CAD build for the part. Positions are in the model's coordinates, mm. A direction names the side the tool comes from. Give positions to 0.01 mm unless a question says otherwise; leave off trailing zeros. Write each loop counter-clockwise with the first axis right and the second up, starting at its lowest first coordinate (ties: lowest second). Pieces come first, ordered by that corner, then holes. Notation, with made-up numbers: (2, 18) - (9, 18) arc R26 ccw to (9, 38) - close; hole circle Ø6 at (0, 85.5). An arc over 180 degrees is marked (long way). Answer as a JSON object with one key per item and string values.
Autodesk Inventor part; units mm, degrees
ref_plane "YZ Plane" through (0, 0, 0) normal (1, 0, 0) x (0, 1, 0)
ref_plane "XZ Plane" through (0, 0, 0) normal (0, 1, 0) x (-1, 0, 0)
ref_plane "XY Plane" through (0, 0, 0) normal (0, 0, 1) x (1, 0, 0)
sketch "Sketch1" plane through (0, 0, 0) normal (0, 1, 0) x (-1, 0, 0)
  line L0 (86.0424, 26.9023) -> (56.0424, 26.9023)
  line L1 (2.5, 83.15) -> (-2.5, 83.15)
  line L2 (2.5, 83.15) -> (2.5, 73.15)
  line L3 (-2.5, 83.15) -> (-2.5, 73.15)
  circle A0 centre (0, 0) radius 90.15
  line L4 (-86.0424, 26.9023) -> (-56.0424, 26.9023)
  line L5 (-56.0424, 26.9023) -> (-56.0424, 36.9023)
  line L6 (-56.0424, 36.9023) -> (-66.0424, 36.9023)
  line L7 (56.0424, 26.9023) -> (56.0424, 36.9023)
  line L8 (56.0424, 36.9023) -> (66.0424, 36.9023)
  line L9 (-17.9658, 43.15) -> (-2.5, 73.15)
  line L10 (17.5, 43.15) -> (2.5, 73.15)
  line L11 (17.5, 43.15) -> (26.4443, 47.6221)
  line L12 (26.4443, 47.6221) -> (13.6803, 73.15)
  line L13 (-17.9658, 43.15) -> (-26.9101, 47.6221)
  line L14 (-26.9101, 47.6221) -> (-13.7498, 73.15)
  arc A1 (66.0424, 36.9023) -> (13.6803, 73.15) centre (4.3796, 3.7706) ccw
  arc A2 (-13.7498, 73.15) -> (-66.0424, 36.9023) centre (-4.3742, 3.7807) ccw
  dimension "d28" = 180.3
  dimension "d1" = 30
  dimension "d20" = 5
  dimension "d21" = 10
  dimension "d22" = 10
  dimension "d29" = 30
  dimension "d30" = 10
  dimension "d31" = 10
  dimension "d32" = 10
  dimension "d33" = 10
  dimension "d37" = 10
  dimension "d38" = 10
  dimension "d39" = 70
  dimension "d40" = 70
extrude "Extrusion1" add sketch "Sketch1" along normal blind 7 contours L0 L7 L8 A1 L12 L11 L10 L2 L1 L3 L9 L13 L14 A2 L6 L5 L4 A0 picked at (-11.4052, 63.15)
sketch "Sketch2" plane through (0, 0, 0) normal (0, -1, 0) x (1, 0, 0)
  circle A0 centre (74.2273, 36.5899) radius 3.35
  circle A1 centre (-74.0777, 36.5899) radius 3.35
  circle A2 centre (-13.319, 81.4854) radius 3.35
  circle A3 centre (13.1694, 81.4854) radius 3.35
  point P0 (0, 0)
  dimension "d43" = 6.7
  dimension "d44" = 6.7
  dimension "d45" = 6.7
  dimension "d46" = 6.7
extrude "Extrusion2" cut sketch "Sketch2" against normal blind 4.7
properties part number "Droplet Launcher 2"
Item 1: Cut at C-C (y = 3). Give the cut face in (x, z).
Entries:
{"outline": "(-86.04, 26.9) - (-56.04, 26.9) - (-56.04, 36.9) - (-66.04, 36.9) arc R70 cw to (-13.68, 73.15) - (-26.44, 47.62) - (-17.5, 43.15) - (-2.5, 73.15) - (-2.5, 83.15) - (2.5, 83.15) - (2.5, 73.15) - (17.97, 43.15) - (26.91, 47.62) - (13.75, 73.15) arc R70 cw to (66.04, 36.9) - (56.04, 36.9) - (56.04, 26.9) - (86.04, 26.9) arc R90.15 ccw to start; hole circle Ø6.7 at (-74.08, 36.59); hole circle Ø6.7 at (-13.32, 81.49); hole circle Ø6.7 at (13.17, 81.49); hole circle Ø6.7 at (74.23, 36.59)"}
Item 2: Probe line 1 (X direction, y = 5.25, z = 68.5) (3 decimals); line 2 (Z direction, x = -14, y = 1); line 3 (X direction, y = 6, z = 65) (3 decimals). List the from-to ranges inside material, lowest first. Write a range as from..to.
Entries:
{"line 1": "-58.607..-31.028, -16.005..-4.825, 4.897..16.147, 31.047..58.607", "line 2": "50.15..72.51, 73.11..78.21, 84.77..89.06", "line 3": "-62.466..-38.306, -17.755..-6.575, 6.702..17.951, 38.318..62.466"}
Item 3: Cut at A-A (z = 53). Give the cut face in (x, y) (3 decimals), and give its area (3 significant figures).
Entries:
{"outline": "(-72.925, 0) - (-54.144, 0) - (-54.144, 7) - (-72.925, 7) - close; (-23.755, 0) - (-12.575, 0) - (-12.575, 7) - (-23.755, 7) - close; (12.888, 0) - (24.138, 0) - (24.138, 7) - (12.888, 7) - close; (54.148, 0) - (72.925, 0) - (72.925, 7) - (54.148, 7) - close", "area": "420 mm2"}
Item 4: Mould opens along X. For faces 4 (the cylindrical face through (1.6, 3.451, 90.136)), 5 (the flat face through (71, 3, 26.902)), 6 (the cylindrical face through (-74.8, 2.32, 33.32)), 7 (the flat face through (13, 4.7, 82)) say: +X half, -X half, draft (parallel to the pull), parting line (faces both ways), or undercut.
Entries:
{"face 4": "parting line", "face 5": "draft", "face 6": "undercut", "face 7": "undercut"}
Item 5: Cut at B-B (x = 74). Give the cut face in (y, z), and give its area (3 significant figures).
Entries:
{"outline": "(0, 26.9) - (7, 26.9) - (7, 51.49) - (0, 51.49) - (0, 39.93) - (4.7, 39.93) - (4.7, 33.25) - (0, 33.25) - close", "area": "141 mm2"}
Item 6: Which spindle directions (+Z, -Z, +X, -X, +Y, -Y) get a long thin tool onto all of the face, cutting with end or side? Do faces 1 (the flat face through (-2.5, 3, 78)), 2 (the flat face through (-61, 3, 36.902)), 3 (the flat face through (74, 4.7, 37)). Say none if no direction does.
Entries:
{"face 1": "-Z, +Y, -Y", "face 2": "+Y, -Y", "face 3": "-Y"}
Item 7: Cut at D-D (z = 63.5). Give the cut face in (x, y) (3 decimals), and give its area (3 significant figures).
Entries:
{"outline": "(-63.99, 0) - (-40.882, 0) - (-40.882, 7) - (-63.99, 7) - close; (-18.505, 0) - (-7.325, 0) - (-7.325, 7) - (-18.505, 7) - close; (7.475, 0) - (18.725, 0) - (18.725, 7) - (7.475, 7) - close; (40.893, 0) - (63.99, 0) - (63.99, 7) - (40.893, 7) - close", "area": "480 mm2"}
Item 8: Flat gauge pins, fed straight in: P1, Ø1.5, axis at y = 4.5, z = 57, coming from the +X side; P2, Ø1.5, axis at y = 5, z = 34.5, coming from the -X side; P3, Ø6, axis at x = -13.32, z = 81.49, coming from the -Y side. Where does each tip first touch, or does it go through?
Entries:
{"P1": "x = 70.45", "P2": "x = -83.59", "P3": "y = 4.7"}
